from build123d import *

# Parameters (mm, degrees)
SKETCH1_W           = 50
SKETCH1_H           = 18
BOSS_EXTRUDE1_DEPTH = 1.5
SKETCH2_R           = 2.5
CUT_EXTRUDE1_DEPTH  = 10
SKETCH3_R           = 0.55
CUT_EXTRUDE2_DEPTH  = 2.5
SKETCH4_R           = 0.55
CUT_EXTRUDE3_DEPTH  = 2.5
SKETCH8_R           = 0.55
CUT_EXTRUDE5_DEPTH  = 2.5
FILLET2_R           = 1


with BuildPart() as part:
    # Sketch1 → Boss-Extrude1 (new body)
    with BuildSketch(Plane(origin=(0, 0, 0), x_dir=(1, 0, 0), z_dir=(0, 1, 0))):
        Rectangle(SKETCH1_W, SKETCH1_H)
    extrude(amount=BOSS_EXTRUDE1_DEPTH)

    # Sketch2 → Cut-Extrude1 (cut)
    with BuildSketch(Plane(origin=(0, 1.5, 0), x_dir=(1, 0, 0), z_dir=(0, 1, 0))):
        with Locations((-15.25, 6.875)):
            Circle(SKETCH2_R)
        with Locations((-0.25, -4.875)):
            Circle(SKETCH2_R)
    extrude(amount=-CUT_EXTRUDE1_DEPTH, mode=Mode.SUBTRACT)

    # Sketch3 → Cut-Extrude2 (cut, through all)
    with BuildSketch(Plane.XZ):
        with Locations((-17, 0)):
            Circle(SKETCH3_R)
        with Locations((-4, 0)):
            Circle(SKETCH3_R)
        with Locations((9, 0)):
            Circle(SKETCH3_R)
        with Locations((-19.54, 0)):
            Circle(SKETCH3_R)
        with Locations((-14.46, 0)):
            Circle(SKETCH3_R)
        with Locations((-6.54, 0)):
            Circle(SKETCH3_R)
        with Locations((-1.46, 0)):
            Circle(SKETCH3_R)
        with Locations((6.46, 0)):
            Circle(SKETCH3_R)
        with Locations((11.54, 0)):
            Circle(SKETCH3_R)
    extrude(amount=-CUT_EXTRUDE2_DEPTH, mode=Mode.SUBTRACT)

    # Sketch4 → Cut-Extrude3 (cut, through all)
    with BuildSketch(Plane(origin=(0, 1.5, 0), x_dir=(1, 0, 0), z_dir=(0, 1, 0))):
        with Locations((19, -2.54)):
            Circle(SKETCH4_R)
        with Locations((19, -5.08)):
            Circle(SKETCH4_R)
        with Locations((19, -7.62)):
            Circle(SKETCH4_R)
        with Locations((19, 2.54)):
            Circle(SKETCH4_R)
        with Locations((19, 5.08)):
            Circle(SKETCH4_R)
        with Locations((19, 7.62)):
            Circle(SKETCH4_R)
        with Locations((16, 0)):
            Circle(SKETCH4_R)
    extrude(amount=-CUT_EXTRUDE3_DEPTH, mode=Mode.SUBTRACT)

    # Sketch8 → Cut-Extrude5 (cut, through all)
    with BuildSketch(Plane(origin=(0, 1.5, 0), x_dir=(1, 0, 0), z_dir=(0, 1, 0))):
        with Locations((-10.756904198, -0.352285973)):
            Circle(SKETCH8_R)
        with Locations((-8.129113164, -6.033080496)):
            Circle(SKETCH8_R)
        with Locations((-19.014042493, -7.62)):
            Circle(SKETCH8_R)
        with Locations((-1.46, 5.08)):
            Circle(SKETCH8_R)
        with Locations((12.244030361, 2.54)):
            Circle(SKETCH8_R)
        with Locations((15.717799533, 5.08)):
            Circle(SKETCH8_R)
    extrude(amount=-CUT_EXTRUDE5_DEPTH, mode=Mode.SUBTRACT)

    # Fillet2
    fillet2_edges = [part.edges().sort_by_distance(p)[0] for p in [
        (-13.933043281, 0.75, -9),
        (-16.566956719, 0.75, -9),
    ]]
    fillet(fillet2_edges, radius=FILLET2_R)


solid = part.part
Read the model definition and answer for the solid it produces. Units are mm, in the model's axes. A direction names the side the tool comes from. Round coordinates to 2 decimals unless told otherwise and drop trailing zeros. Loops run counter-clockwise (first coordinate to the right, second up) from the corner with the lowest first, then second, coordinate; pieces in that order, holes last. Notation, with made-up numbers: (22, 68.5) - (44, 68.5) arc R24 ccw to (44, 103.5) - close; hole circle Ø11 at (73.5, 84.5). An arc over 180 degrees is marked (long way). One line per question, with ' | ' between items. Start each with the question number.
Q1. Section C-C on y = 1.15 is taken. Count the separate pieces of the cut face and the enclosed holes in it, plus the area to 3 significant figures.
Q2. Section B-B on z = -6.5 is taken. Give the vertices of the cut face in (x, y), plus the area to 3 significant figures.
Q3. Section A-A on x = 6.46 is taken. Give the vertices of the cut face in (y, z), plus the area to 4 significant figures.
Q4. Find the intervals of material crossed by L1, parallel to Z at x = 11.5, y = 0.7; L2, parallel to X at y = 0.35, z = -8; L3, parallel to X at y = 0.75, z = 6.25, in increasing order.
Q5. For a pull along Z with two mould halves and no side action, classify faces 1 (the cylindrical face through (-16.475, 0.74, 0.165)), 2 (the flat face through (-22, 1, -9)), 3 (the flat face through (0, 1, 9)) as +Z half, -Z half, draft (parallel to the pull), parting line (faces both ways), or undercut.
Q6. A flat-ended cylindrical pin translates along its axis: pin 1 (0.7 mm diameter, centred on x = 19, z = 7.62, fed in from +Y). Find the tip coordinate at first contact, or state that the pin passes through.
Q7. For faces 4 (the flat face through (0, 0, 0)), 5 (the cylindrical face through (-12.756, 0.76, -8.572)), determine the directions among +Z, -Z, +X, -X, +Y, -Y from which every point of the face is accessible in a straight line to the end or side of a thin tool.
Established:
1) separate pieces: 1 | enclosed holes: 23 | area: 839 mm²
2) outline: (-25, 0) - (-17.72, 0) - (-17.72, 1.5) - (-25, 1.5) - close; (-12.78, 0) - (25, 0) - (25, 1.5) - (-12.78, 1.5) - close | area: 67.6 mm²
3) outline: (0, -9) - (1.5, -9) - (1.5, -0.55) - (0, -0.55) - close; (0, 0.55) - (1.5, 0.55) - (1.5, 9) - (0, 9) - close | area: 25.35 mm²
4) L1: -9 to -0.55, 0.55 to 9 | L2: -25 to -17.56, -12.94 to 18.6, 19.4 to 25 | L3: -25 to -8.63, -7.62 to -2.34, 1.84 to 25
5) face 1: undercut | face 2: -Z half | face 3: +Z half
6) pin 1: through
7) face 4: +Z, -Z, +X, -X, -Y | face 5: +Y, -Y
